Source: three-view drawing plus pictorial views. Frame: mm from the lowest corner of the part. A direction names the side the tool comes from. Round coordinates to 2 decimals unless told otherwise and drop trailing zeros. Write each loop counter-clockwise with the first axis right and the second up, starting at its lowest first coordinate (ties: lowest second). Pieces come first, ordered by that corner, then holes. Notation, with made-up numbers: M 16,-4.5 L 33,-4.5 A28 ccw 33,18.5 Z; hole C 75,42.5 d11. An arc over 180 degrees is marked long. Answer in a Markdown table with one row per item.
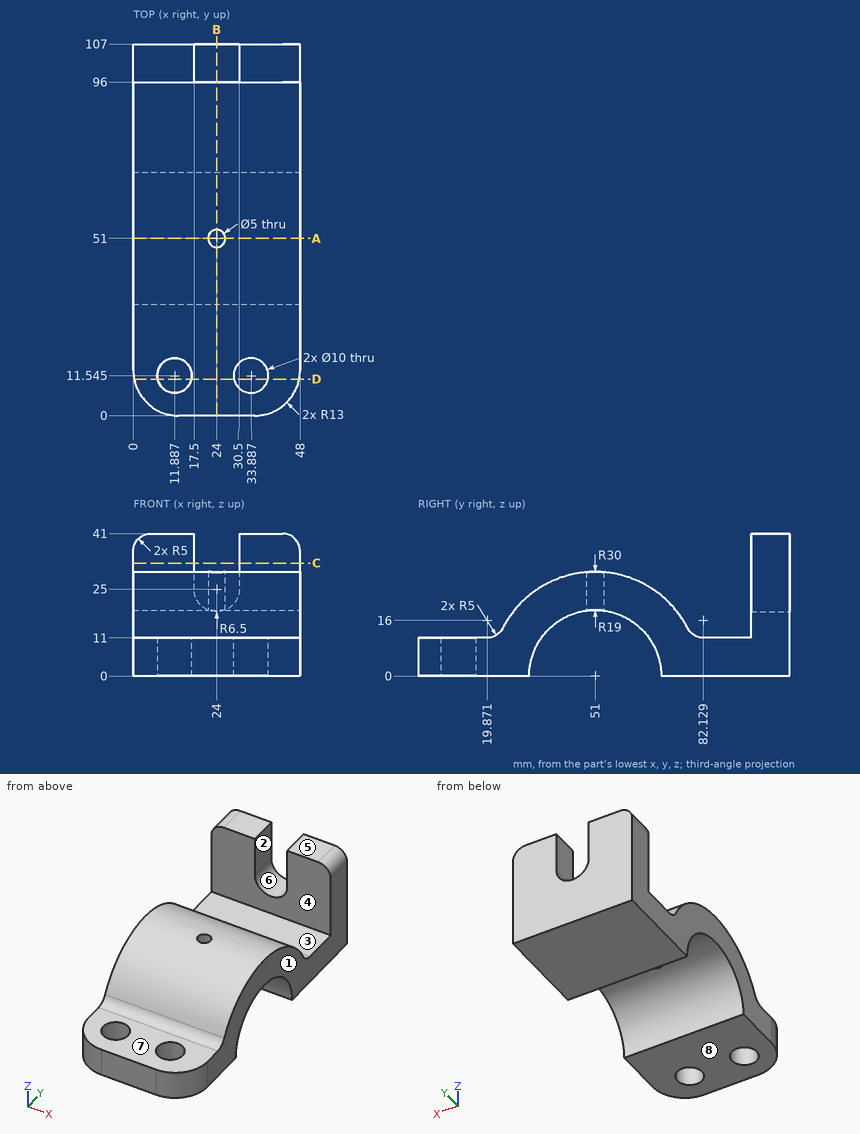
Q1. Contact query for flat-ended pins moving along their axis: pin 1 Ø6 at (x, y) = (38.5, 45.5) entering from +Z; pin 2 Ø2 at (x, y) = (18.5, 80) entering from +Z; pin 3 Ø1 at (x, z) = (19.5, 35.5) entering from -Y; pin 4 Ø1.5 at (x, y) = (12.5, 64) entering from -Z. Output: stop coordinate, or through.
Solutions:
| item | result |
|---|---|
| pin 1 | stops at z = 29.9 |
| pin 2 | stops at z = 12.1 |
| pin 3 | passes through |
| pin 4 | stops at z = 13.11 |
Q2. Pull-direction query (X, two-part tool) for the marked faces 1, 2 and 3; classes: pulls with the +X half, pulls with the -X half, needs draft (parallel to the pull), parting line crosses it, or undercut.
Solutions:
| item | result |
|---|---|
| face 1 | pulls with the +X half |
| face 2 | undercut |
| face 3 | needs draft |
Q3. Section D-D (y = 10.5). Return loops of the section in (x, z).
Solutions:
| item | result |
|---|---|
| outline | M 0.24,0 L 7,0 L 7,11 L 0.24,11 Z; M 16.78,0 L 29,0 L 29,11 L 16.78,11 Z; M 38.78,0 L 47.76,0 L 47.76,11 L 38.78,11 Z |
Q4. Section C-C (z = 32.5). Return loops of the section in (x, y).
Solutions:
| item | result |
|---|---|
| outline | M 0,96 L 17.5,96 L 17.5,107 L 0,107 Z; M 30.5,96 L 48,96 L 48,107 L 30.5,107 Z |
Q5. Section B-B (x = 24). Return loops of the section in (y, z) (1 decimal).
Solutions:
| item | result |
|---|---|
| outline | M 0,0 L 32,0 A19 cw 48.5,18.8 L 48.5,29.9 A30 ccw 24.3,13.7 A5 cw 19.9,11 L 0,11 Z; M 53.5,18.8 A19 cw 70,0 L 107,0 L 107,18.5 L 96,18.5 L 96,11 L 82.1,11 A5 cw 77.7,13.7 A30 ccw 53.5,29.9 Z |
Q6. Section A-A (y = 51). Return loops of the section in (x, z), and give its area (3 significant figures).
Solutions:
| item | result |
|---|---|
| outline | M 0,19 L 21.5,19 L 21.5,30 L 0,30 Z; M 26.5,19 L 48,19 L 48,30 L 26.5,30 Z |
| area | 473 mm2 |
Q7. Access query for the marked faces 4, 5, 6, 7 and 8. Directions: +Z, -Z, +X, -X, +Y, -Y. A direction counts if a zero-diameter tool reaches every point of the face in a straight line with its end or side. Return the directions, or none.
Solutions:
| item | result |
|---|---|
| face 4 | +Z, +X, -X |
| face 5 | +Z, +X, -X, +Y, -Y |
| face 6 | +Z, +Y |
| face 7 | +Z, +X, -X, -Y |
| face 8 | -Z, +X, -X, +Y, -Y |
Q8. Material intervals for probe 1 along Y at (x, z) = (19, 14) (1 decimal); probe 2 along Y at (x, z) = (32.5, 33.5); probe 3 along Z at (x, y) = (26.5, 5), sorted ascending.
Solutions:
| item | result |
|---|---|
| probe 1 | y = 24.5 to 38.2, 63.8 to 77.5, 96 to 107 |
| probe 2 | y = 96 to 107 |
| probe 3 | z = 0 to 11 |
